```python
from build123d import *

# Parameters (mm, degrees)
MODEL_W                 = 3
MODEL_H                 = 3
SALIENTE_EXTRUIR1_DEPTH = 3


with BuildPart() as part:
    # Model → Saliente-Extruir1 (new body)
    with BuildSketch(Plane.XY):
        with BuildLine():
            Line((9.821574141, 299.540447034), (18.821574141, 299.540447034))
            ThreePointArc((18.821574141, 299.540447034), (22.003554656, 298.222427549), (23.321574141, 295.040447034))
            Line((23.321574141, 295.040447034), (23.321574141, 286.040447034))
            ThreePointArc((23.321574141, 286.040447034), (22.003554656, 282.858466518), (18.821574141, 281.540447034))
            Line((18.821574141, 281.540447034), (9.821574141, 281.540447034))
            ThreePointArc((9.821574141, 281.540447034), (6.639593626, 282.858466518), (5.321574141, 286.040447034))
            Line((5.321574141, 286.040447034), (5.321574141, 295.040447034))
            ThreePointArc((5.321574141, 295.040447034), (6.639593626, 298.222427549), (9.821574141, 299.540447034))
        make_face()
        with Locations((9.821574141, 295.040447034)):
            Rectangle(MODEL_W, MODEL_H, mode=Mode.SUBTRACT)
        with Locations((18.821574141, 295.040447034)):
            Rectangle(MODEL_W, MODEL_H, mode=Mode.SUBTRACT)
        with Locations((9.821574141, 286.040447034)):
            Rectangle(MODEL_W, MODEL_H, mode=Mode.SUBTRACT)
        with Locations((18.821574141, 286.040447034)):
            Rectangle(MODEL_W, MODEL_H, mode=Mode.SUBTRACT)
    extrude(amount=SALIENTE_EXTRUIR1_DEPTH)


solid = part.part
```
Source: CAD feature listing. Evaluate the final solid. Frame: model axes, mm. A direction names the side the tool comes from. Coordinates: 2 decimals unless noted, no trailing zeros. Loops run counter-clockwise (first coordinate to the right, second up) from the corner with the lowest first, then second, coordinate; pieces in that order, holes last. Notation, with made-up numbers: M 77.25,42 L 89.25,42 A8 cw 89.25,50 Z; hole C -30.75,72 d2. An arc over 180 degrees is marked long. Put each result on its own line as item: value. Start each with the question number.
1) Cut plane B-B on y = 284.75. Return the cut outline in (x, z), then the cut area to 3 significant figures.
2) Cut plane A-A on x = 10.75. Return the cut outline in (y, z).
3) Ray query, L1, parallel to X at y = 295, z = 2.6; L2, parallel to Y at x = 11.25, z = 2.55; L3, parallel to Y at x = 9.25, z = 0.85. Return the intervals inside material, ascending. Write a range as from..to.
4) Cut plane D-D on x = 21.5. Return the cut outline in (y, z).
5) Cut plane C-C on z = 2.45. Return the cut outline in (x, y), then the cut area to 3 significant figures.
6) Contact query for a flat-ended pin moving along its axis: pin 1 Ø0.9 at (x, z) = (9, 2) entering from -Y. Output: stop coordinate, or through.
7) Reachability of faces 1 (the face through (21.968, 298.257, 1.479)), 2 (the face through (11.322, 295, 1)) from +Z, -Z, +X, -X, +Y, -Y: full face, straight path, thin tool, end or side. Return the list, or none.
8) Pull-direction query (X, two-part tool) for faces 3 (the face through (10, 296.54, 1)), 4 (the face through (14, 299.54, 1)), 5 (the face through (19, 293.54, 1)), 6 (the face through (5.322, 290, 1)); classes: pulls with the +X half, pulls with the -X half, needs draft (parallel to the pull), parting line crosses it, or undercut.
The answers:
1. outline: M 5.51,0 L 8.32,0 L 8.32,3 L 5.51,3 Z; M 11.32,0 L 17.32,0 L 17.32,3 L 11.32,3 Z; M 20.32,0 L 23.13,0 L 23.13,3 L 20.32,3 Z
1. area: 34.9 mm²
2. outline: M 281.54,0 L 284.54,0 L 284.54,3 L 281.54,3 Z; M 287.54,0 L 293.54,0 L 293.54,3 L 287.54,3 Z; M 296.54,0 L 299.54,0 L 299.54,3 L 296.54,3 Z
3. L1: x = 5.32..8.32, 11.32..17.32, 20.32..23.32
3. L2: y = 281.54..284.54, 287.54..293.54, 296.54..299.54
3. L3: y = 281.58..284.54, 287.54..293.54, 296.54..299.5
4. outline: M 282.42,0 L 298.66,0 L 298.66,3 L 282.42,3 Z
5. outline: M 5.32,286.04 A4.5 ccw 9.82,281.54 L 18.82,281.54 A4.5 ccw 23.32,286.04 L 23.32,295.04 A4.5 ccw 18.82,299.54 L 9.82,299.54 A4.5 ccw 5.32,295.04 Z; hole M 8.32,284.54 L 11.32,284.54 L 11.32,287.54 L 8.32,287.54 Z; hole M 8.32,293.54 L 11.32,293.54 L 11.32,296.54 L 8.32,296.54 Z; hole M 17.32,284.54 L 20.32,284.54 L 20.32,287.54 L 17.32,287.54 Z; hole M 17.32,293.54 L 20.32,293.54 L 20.32,296.54 L 17.32,296.54 Z
5. area: 271 mm²
6. pin 1: stops at y = 281.56
7. face 1: +Z, -Z, +X, +Y
7. face 2: +Z, -Z
8. face 3: undercut
8. face 4: needs draft
8. face 5: undercut
8. face 6: pulls with the -X half
